The model under review builds one solid part; all positions refer to its coordinate system, in mm. Face numbers are marked on the shaded views. Round coordinates to 2 decimals unless told otherwise and drop trailing zeros. Write each loop counter-clockwise with the first axis right and the second up, starting at its lowest first coordinate (ties: lowest second). Pieces come first, ordered by that corner, then holes. Notation, with made-up numbers: (25.25, -26.75) - (43.25, -26.75) arc R22 ccw to (43.25, 11.25) - close; hole circle Ø10 at (78.5, 42.25). An arc over 180 degrees is marked (long way). Use one line per item in the form item = value.
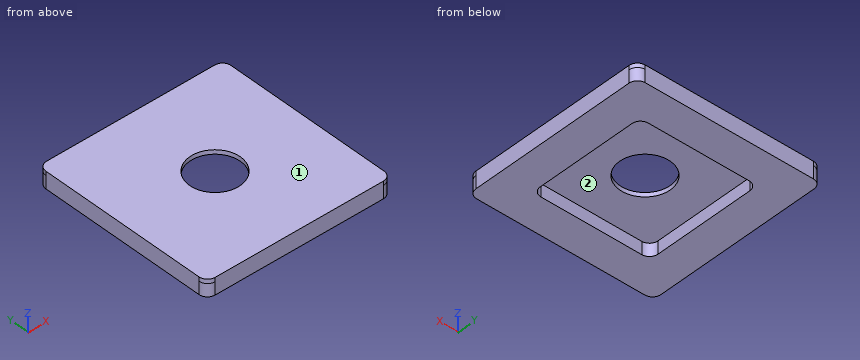
from build123d import *

# Parameters (mm, degrees)
F0_W     = 11
F0_H     = 11
F0_W_2   = 7
F0_H_2   = 7
F1_DEPTH = 0.75
F2_R     = 0.5
F4_DEPTH = 0.25
F5_R     = 1.5
F6_DEPTH = 1.001


with BuildPart() as f1:
    # F0 (on Top) → F1 (new body)
    with BuildSketch(Plane.XY):
        with Locations((3.5, 3.5)):
            Rectangle(F0_W, F0_H)
        with Locations((3.5, 3.5)):
            Rectangle(F0_W_2, F0_H_2, mode=Mode.SUBTRACT)
    extrude(amount=F1_DEPTH)

    # F2
    f2_edges = [f1.edges().sort_by_distance(p)[0] for p in [
        (0, 7, 0.375),
        (7, 7, 0.375),
        (9, 9, 0.375),
        (-2, 9, 0.375),
        (-2, -2, 0.375),
        (9, -2, 0.375),
        (0, 0, 0.375),
        (7, 0, 0.375),
    ]]
    fillet(f2_edges, radius=F2_R)

    # F3 (on face) → F4 (join)
    with BuildSketch(Plane.XY.offset(0.75)):
        with BuildLine():
            ThreePointArc((-2, -1.5), (-1.8535533906, -1.8535533906), (-1.5, -2))
            Line((-1.5, -2), (8.5, -2))
            ThreePointArc((8.5, -2), (8.8535533906, -1.8535533906), (9, -1.5))
            Line((9, -1.5), (9, 8.5))
            ThreePointArc((9, 8.5), (8.8535533906, 8.8535533906), (8.5, 9))
            Line((8.5, 9), (-1.5, 9))
            ThreePointArc((-1.5, 9), (-1.8535533906, 8.8535533906), (-2, 8.5))
            Line((-2, 8.5), (-2, -1.5))
        make_face()
        with BuildLine():
            ThreePointArc((7, 0.5), (6.8535533906, 0.1464466094), (6.5, 0))
            Line((6.5, 0), (0.5, 0))
            ThreePointArc((0.5, 0), (0.1464466094, 0.1464466094), (0, 0.5))
            Line((0, 0.5), (0, 6.5))
            ThreePointArc((0, 6.5), (0.1464466094, 6.8535533906), (0.5, 7))
            Line((0.5, 7), (6.5, 7))
            ThreePointArc((6.5, 7), (6.8535533906, 6.8535533906), (7, 6.5))
            Line((7, 6.5), (7, 0.5))
        make_face(mode=Mode.SUBTRACT)
        with BuildLine():
            Line((0.5, 0), (6.5, 0))
            ThreePointArc((6.5, 0), (6.8535533906, 0.1464466094), (7, 0.5))
            Line((7, 0.5), (7, 6.5))
            ThreePointArc((7, 6.5), (6.8535533906, 6.8535533906), (6.5, 7))
            Line((6.5, 7), (0.5, 7))
            ThreePointArc((0.5, 7), (0.1464466094, 6.8535533906), (0, 6.5))
            Line((0, 6.5), (0, 0.5))
            ThreePointArc((0, 0.5), (0.1464466094, 0.1464466094), (0.5, 0))
        make_face()
    extrude(amount=F4_DEPTH)

    # F5 (on face) → F6 (cut, through all)
    with BuildSketch(Plane.XY.offset(1)):
        with Locations((3.5, 3.5)):
            Circle(F5_R)
    extrude(amount=-F6_DEPTH, mode=Mode.SUBTRACT)


solid = f1.part
(1) Add section A-A on y = 3.5. Write out the cut boundary in (x, z), then the cut area to 3 significant figures.
Geometry results:
outline = (-2, 0) - (0, 0) - (0, 0.75) - (2, 0.75) - (2, 1) - (-2, 1) - close; (5, 0.75) - (7, 0.75) - (7, 0) - (9, 0) - (9, 1) - (5, 1) - close
area = 5.00 mm2
(2) Add section C-C on z = 0.2. Write out the cut boundary in (x, y).
Geometry results:
outline = (-2, -1.5) arc R0.5 ccw to (-1.5, -2) - (8.5, -2) arc R0.5 ccw to (9, -1.5) - (9, 8.5) arc R0.5 ccw to (8.5, 9) - (-1.5, 9) arc R0.5 ccw to (-2, 8.5) - close; hole (0, 0.5) arc R0.5 ccw to (0.5, 0) - (6.5, 0) arc R0.5 ccw to (7, 0.5) - (7, 6.5) arc R0.5 ccw to (6.5, 7) - (0.5, 7) arc R0.5 ccw to (0, 6.5) - close
(3) Add section D-D on y = 6. Write out the cut boundary in (x, z).
Geometry results:
outline = (-2, 0) - (0, 0) - (0, 0.75) - (7, 0.75) - (7, 0) - (9, 0) - (9, 1) - (-2, 1) - close
(4) To check wall thickness, follow L1, parallel to X at y = 1, z = 0.25; L2, parallel to Y at x = 3.5, z = 0.95. State the ranges of each line that lie inside material, in increasing order.
Geometry results:
L1 = -2 to 0, 7 to 9
L2 = -2 to 2, 5 to 9
(5) The part is to be moulded in two halves that separate along X. For the marked faces 1 and 2, say which applies: +X half, -X half, draft (parallel to the pull), parting line (faces both ways), or undercut.
Geometry results:
face_1 = draft
face_2 = undercut
